Here's how the part is built. I have some questions about the finished solid (model axes, mm). A direction names the side the tool comes from. Round coordinates to 2 decimals unless told otherwise and drop trailing zeros. Loops run counter-clockwise (first coordinate to the right, second up) from the corner with the lowest first, then second, coordinate; pieces in that order, holes last. Notation, with made-up numbers: M -14.75,-29.75 L -4.75,-29.75 A29 cw -4.75,1.25 Z; hole C 35,41 d9. An arc over 180 degrees is marked long. Use a Markdown table: item, result.
```python
from build123d import *

# Parameters (mm, degrees)
CROQUIS1_W              = 20
CROQUIS1_H              = 20
SALIENTE_EXTRUIR1_DEPTH = 2
CROQUIS2_W              = 4
CROQUIS2_H              = 16
SALIENTE_EXTRUIR2_DEPTH = 5
CORTAR_EXTRUIR2_DEPTH   = 5
CORTAR_EXTRUIR3_START   = -5
CORTAR_EXTRUIR3_DEPTH   = 5
REDONDEO1_R             = 2
REDONDEO2_R             = 2


with BuildPart() as part:
    # Croquis1 → Saliente-Extruir1 (new body)
    with BuildSketch(Plane(origin=(0, 0, 0), x_dir=(1, 0, 0), z_dir=(0, 1, 0))):
        with Locations((-2.554744526, 1.751824818)):
            Rectangle(CROQUIS1_W, CROQUIS1_H)
    extrude(amount=SALIENTE_EXTRUIR1_DEPTH)

    # Croquis2 → Saliente-Extruir2 (add)
    with BuildSketch(Plane(origin=(0, 2, 0), x_dir=(1, 0, 0), z_dir=(0, 1, 0))):
        with Locations((-10.554744526, 1.751824818)):
            Rectangle(CROQUIS2_W, CROQUIS2_H)
        with Locations((5.445255474, 1.751824818)):
            Rectangle(CROQUIS2_W, CROQUIS2_H)
    extrude(amount=SALIENTE_EXTRUIR2_DEPTH)

    # Croquis3 → Cortar-Extruir2 (cut)
    with BuildSketch(Plane(origin=(-8.554744526, 0, 0), x_dir=(0, 0, -1), z_dir=(1, 0, 0))):
        with BuildLine():
            Line((6.251824818, 4.5), (-2.748175182, 4.5))
            ThreePointArc((-2.748175182, 4.5), (-3.455281964, 4.207106781), (-3.748175182, 3.5))
            Line((-3.748175182, 3.5), (-3.748175182, 2.5))
            Line((-3.748175182, 2.5), (7.251824818, 2.5))
            Line((7.251824818, 2.5), (7.251824818, 3.5))
            ThreePointArc((7.251824818, 3.5), (6.958931599, 4.207106781), (6.251824818, 4.5))
        make_face()
    extrude(amount=-CORTAR_EXTRUIR2_DEPTH, mode=Mode.SUBTRACT)

    # Croquis4 → Cortar-Extruir3 (cut)
    with BuildSketch(Plane.ZY.offset(-3.445255474).offset(CORTAR_EXTRUIR3_START)):
        with BuildLine():
            Line((2.748175182, 4.5), (-6.251824818, 4.5))
            ThreePointArc((-6.251824818, 4.5), (-6.958931599, 4.207106781), (-7.251824818, 3.5))
            Line((-7.251824818, 3.5), (-7.251824818, 2.5))
            Line((-7.251824818, 2.5), (3.748175182, 2.5))
            Line((3.748175182, 2.5), (3.748175182, 3.5))
            ThreePointArc((3.748175182, 3.5), (3.455281964, 4.207106781), (2.748175182, 4.5))
        make_face()
    extrude(amount=CORTAR_EXTRUIR3_DEPTH, mode=Mode.SUBTRACT)

    # Redondeo1
    redondeo1_edges = [part.edges().sort_by_distance(p)[0] for p in [
        (7.445255474, 1, -11.751824818),
        (-12.554744526, 1, -11.751824818),
        (7.445255474, 1, 8.248175182),
        (-12.554744526, 1, 8.248175182),
    ]]
    fillet(redondeo1_edges, radius=REDONDEO1_R)

    # Redondeo2
    redondeo2_edges = [part.edges().sort_by_distance(p)[0] for p in [
        (5.445255474, 7, -9.751824818),
        (5.445255474, 7, 6.248175182),
        (-10.554744526, 7, -9.751824818),
        (-10.554744526, 7, 6.248175182),
    ]]
    fillet(redondeo2_edges, radius=REDONDEO2_R)


solid = part.part
```
Q1. Will these pins go through, and if not, where does the flat tip stop? P1, Ø3.5, axis at x = 4.5, y = 4, coming from the -Z side; P2, Ø1, axis at x = 1, y = 5, coming from the +Z side; P3, Ø2, axis at x = 5, z = -3.5, coming from the -Y side; P4, Ø0.5, axis at x = 5.5, y = 3, coming from the +Z side.
Return value:
| item | result |
|---|---|
| P1 | stops at z = -9.75 |
| P2 | passes through |
| P3 | stops at y = 0 |
| P4 | stops at z = 6.25 |
Q2. We'd pull the mould along Z, two halves only. Please class faces 4 (the cylindrical face through (-10.527, 6.399, 5.678)), 5 (the flat face through (-3, 2, -2)), 6 (the flat face through (5, 3, -7.252)): pulls with the +Z half, pulls with the -Z half, needs draft (parallel to the pull), parting line crosses it, or undercut.
Return value:
| item | result |
|---|---|
| face 4 | pulls with the +Z half |
| face 5 | needs draft |
| face 6 | undercut |
Q3. Imagine slicing it at C-C, the plane x = 5. Please give me the cut outline in (y, z), then the cut area to 3 significant figures.
Return value:
| item | result |
|---|---|
| outline | M 0,-11.75 L 2,-11.75 L 2,-9.75 L 5,-9.75 A2 ccw 7,-7.75 L 7,4.25 A2 ccw 5,6.25 L 2,6.25 L 2,8.25 L 0,8.25 Z; hole M 2.5,-7.25 L 3.5,-7.25 A1 ccw 4.5,-6.25 L 4.5,2.75 A1 ccw 3.5,3.75 L 2.5,3.75 Z |
| area | 96.7 mm^2 |
Q4. Imagine slicing it at B-B, the plane z = 0.75. Please give me the cut outline in (x, y).
Return value:
| item | result |
|---|---|
| outline | M -12.55,0 L 7.45,0 L 7.45,2.5 L 3.45,2.5 L 3.45,2 L -8.55,2 L -8.55,2.5 L -12.55,2.5 Z; M -12.55,4.5 L -8.55,4.5 L -8.55,7 L -12.55,7 Z; M 3.45,4.5 L 7.45,4.5 L 7.45,7 L 3.45,7 Z |
Q5. I need wall thicknesses on line 1 (Z direction, x = 5, y = 3.5); line 2 (X direction, y = 4.5, z = -9.5); line 3 (Y direction, x = -6.5, z = -5). Which ranges of each line are inside material? Lowest first, please. Write a range as from..to.
Return value:
| item | result |
|---|---|
| line 1 | z = -9.75..-7.25, 3.75..6.25 |
| line 2 | x = -12.55..-8.55, 3.45..7.45 |
| line 3 | y = 0..2 |
Q6. Imagine slicing it at D-D, the plane z = -9.25. Please give me the cut outline in (x, y).
Return value:
| item | result |
|---|---|
| outline | M -12.55,0 L 7.45,0 L 7.45,6.32 L 3.45,6.32 L 3.45,2 L -8.55,2 L -8.55,6.32 L -12.55,6.32 Z |
Q7. For faces 1 (the flat face through (-11, 4.5, -2)), 2 (the flat face through (-11, 3, 6.248)), 3 (the flat face through (-11, 3, -9.752)), which set-ups out of +Z, -Z, +X, -X, +Y, -Y let a thin tool reach every point of the face, with its end or its side?
Return value:
| item | result |
|---|---|
| face 1 | +X, -X |
| face 2 | +Z, +X, -X, +Y |
| face 3 | -Z, +X, -X, +Y |
Q8. Imagine slicing it at A-A, the plane y = 4.75. Please give me the cut outline in (x, z), then the cut area to 3 significant figures.
Return value:
| item | result |
|---|---|
| outline | M -12.55,-9.75 L -8.55,-9.75 L -8.55,6.25 L -12.55,6.25 Z; M 3.45,-9.75 L 7.45,-9.75 L 7.45,6.25 L 3.45,6.25 Z |
| area | 128 mm^2 |
